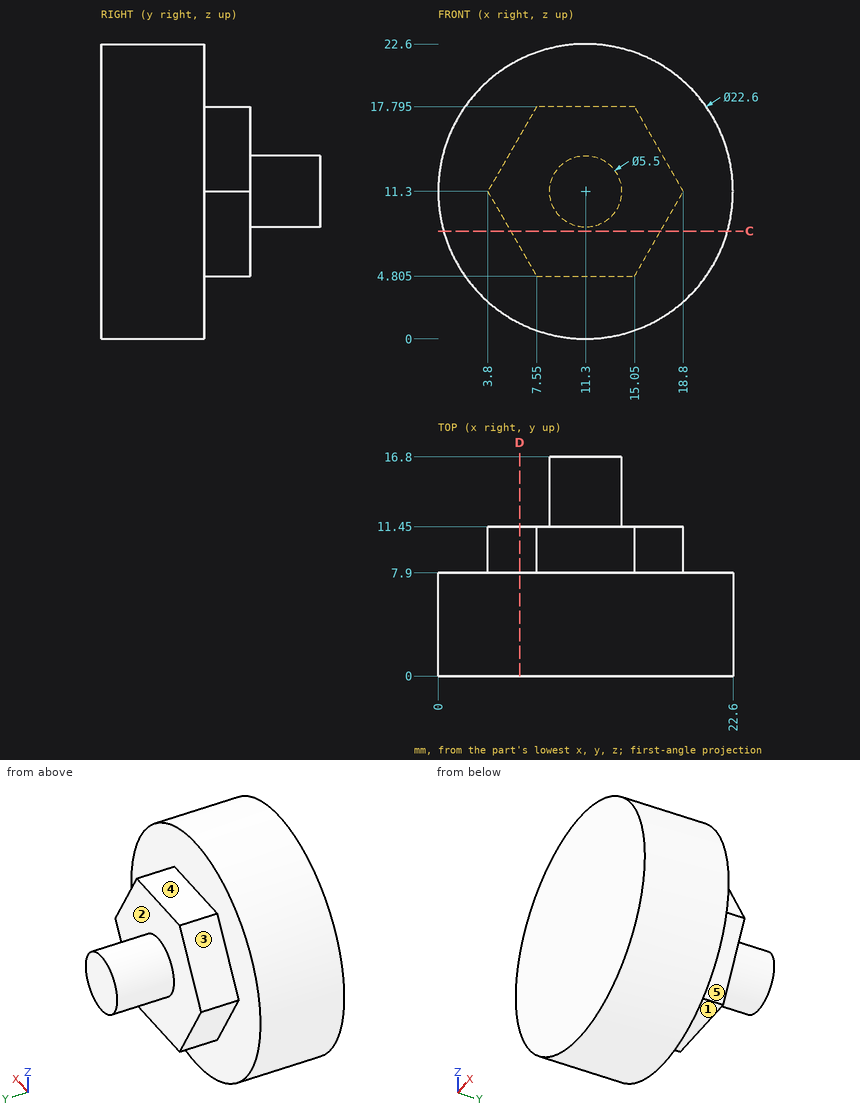
Design review of the part shown in the three views and the two pictorial views. Dimensions are in mm from the part's minimum x, y and z. A direction names the side the tool comes from. Round coordinates to 2 decimals unless told otherwise and drop trailing zeros. Loops run counter-clockwise (first coordinate to the right, second up) from the corner with the lowest first, then second, coordinate; pieces in that order, holes last. Notation, with made-up numbers: (56, 66.25) - (78, 66.25) arc R29 cw to (78, 90.25) - close; hole circle Ø4 at (2.25, 2.25). An arc over 180 degrees is marked (long way). Answer as CSV lines item,"result".
(1) Consider section D-D on x = 6.25. Give the boundary of the cut face in (y, z).
Checked values:
outline,"(0, 1.19) - (7.9, 1.19) - (7.9, 7.06) - (11.45, 7.06) - (11.45, 15.54) - (7.9, 15.54) - (7.9, 21.41) - (0, 21.41) - close"
(2) Consider section C-C on z = 8.25. Give the boundary of the cut face in (x, y), then the cut area to 3 significant figures.
Checked values:
outline,"(0.42, 0) - (22.18, 0) - (22.18, 7.9) - (17.04, 7.9) - (17.04, 11.45) - (5.56, 11.45) - (5.56, 7.9) - (0.42, 7.9) - close"
area,"213 mm2"
(3) Wall thickness on line 1 (Y direction, x = 15.25, z = 9); line 2 (Y direction, x = 1.5, z = 8.5); line 3 (Z direction, x = 10.75, y = 8.5) (1 decimal): over which ranges is each line inside the solid? List them lowest first.
Checked values:
line 1,"y = 0 to 11.45"
line 2,"y = 0 to 7.9"
line 3,"z = 4.8 to 17.8"
(4) Tool access review of the marked faces 1, 2, 3, 4 and 5: name each direction out of +Z, -Z, +X, -X, +Y, -Y from which nothing blocks a thin tool from reaching the whole face with its end or side.
Checked values:
face 1,"-Z, +X, -X, +Y"
face 2,"+Y"
face 3,"+Z, -X, +Y"
face 4,"+Z, +X, -X, +Y"
face 5,"-Z, +X, +Y"
(5) Insertion check: P1, Ø8, axis at x = 5.5, z = 5.5, coming from the +Y side; P2, Ø3, axis at x = 4, y = 11.5, coming from the -Z side; P3, Ø3, axis at x = 6, y = 5, coming from the +Z side. Each pin has a flat end and moves straight along its axis. Give the tip position at first contact, or say it passes through.
Checked values:
P1,"stops at y = 11.45"
P2,"stops at z = 8.36"
P3,"stops at z = 21.94"
